from build123d import *

# Parameters (mm, degrees)
BOSS_EXTRUDE1_DEPTH = 28
SKETCH2_W           = 1
SKETCH2_H           = 2
BOSS_EXTRUDE2_DEPTH = 28
SKETCH3_W           = 1
SKETCH3_H           = 2
CUT_EXTRUDE1_DEPTH  = 60.264016753
SKETCH4_R           = 7.5
CUT_EXTRUDE2_DEPTH  = 10
SKETCH5_W           = 1
SKETCH5_H           = 2
CUT_EXTRUDE3_DEPTH  = 10
SKETCH6_W           = 7
SKETCH6_H           = 7.5
CUT_EXTRUDE4_DEPTH  = 2
SKETCH7_W           = 7
SKETCH7_H           = 18.5
CUT_EXTRUDE5_DEPTH  = 1


with BuildPart() as part:
    # Sketch1 → Boss-Extrude1 (new body)
    with BuildSketch(Plane.XY):
        with BuildLine():
            Line((-30.589041096, 0), (-30.589041096, 33))
            ThreePointArc((-30.589041096, 33), (-29.124575002, 36.535533906), (-25.589041096, 38))
            Line((-25.589041096, 38), (19.910958904, 38))
            ThreePointArc((19.910958904, 38), (23.44649281, 36.535533906), (24.910958904, 33))
            Line((24.910958904, 33), (24.910958904, 0))
            Line((24.910958904, 0), (24.910958904, -6))
            Line((24.910958904, -6), (26.910958904, -6))
            Line((26.910958904, -6), (26.910958904, 0))
            Line((26.910958904, 0), (26.910958904, 33))
            ThreePointArc((26.910958904, 33), (24.860706372, 37.949747468), (19.910958904, 40))
            Line((19.910958904, 40), (-25.589041096, 40))
            ThreePointArc((-25.589041096, 40), (-30.538788564, 37.949747468), (-32.589041096, 33))
            Line((-32.589041096, 33), (-32.589041096, 0))
            Line((-32.589041096, 0), (-32.589041096, -6))
            Line((-32.589041096, -6), (-30.589041096, -6))
            Line((-30.589041096, -6), (-30.589041096, 0))
        make_face()
    extrude(amount=BOSS_EXTRUDE1_DEPTH)

    # Sketch2 → Boss-Extrude2 (add, through all)
    with BuildSketch(Plane.XY.offset(28)):
        with Locations((-33.089041096, -5)):
            Rectangle(SKETCH2_W, SKETCH2_H)
        with Locations((27.410958904, -5)):
            Rectangle(SKETCH2_W, SKETCH2_H)
    extrude(amount=-BOSS_EXTRUDE2_DEPTH)

    # Sketch3 → Cut-Extrude1 (cut, through all)
    with BuildSketch(Plane.XY.offset(28)):
        with Locations((-32.089041096, -3)):
            Rectangle(SKETCH3_W, SKETCH3_H)
        with Locations((26.410958904, -3)):
            Rectangle(SKETCH3_W, SKETCH3_H)
    extrude(amount=-CUT_EXTRUDE1_DEPTH, mode=Mode.SUBTRACT)

    # Sketch4 → Cut-Extrude2 (cut)
    with BuildSketch(Plane(origin=(0, 40, 0), x_dir=(1, 0, 0), z_dir=(0, 1, 0))):
        with Locations(Location((4.410958904, -11.6, 0), (0, 0, 270))):
            Circle(SKETCH4_R)
    extrude(amount=-CUT_EXTRUDE2_DEPTH, mode=Mode.SUBTRACT)

    # Sketch5 → Cut-Extrude3 (cut)
    with BuildSketch(Plane(origin=(0, 0, 0), x_dir=(-1, 0, 0), z_dir=(0, 0, -1))):
        with Locations((-27.410958904, -5)):
            Rectangle(SKETCH5_W, SKETCH5_H)
    extrude(amount=-CUT_EXTRUDE3_DEPTH, mode=Mode.SUBTRACT)

    # Sketch6 → Cut-Extrude4 (cut)
    with BuildSketch(Plane(origin=(0, 40, 0), x_dir=(1, 0, 0), z_dir=(0, 1, 0))):
        with Locations((-16.089041096, -5.75)):
            Rectangle(SKETCH6_W, SKETCH6_H)
    extrude(amount=-CUT_EXTRUDE4_DEPTH, mode=Mode.SUBTRACT)

    # Sketch7 → Cut-Extrude5 (cut)
    with BuildSketch(Plane(origin=(0, 40, 0), x_dir=(1, 0, 0), z_dir=(0, 1, 0))):
        with Locations((-16.089041096, -18.75)):
            Rectangle(SKETCH7_W, SKETCH7_H)
    extrude(amount=-CUT_EXTRUDE5_DEPTH, mode=Mode.SUBTRACT)


solid = part.part
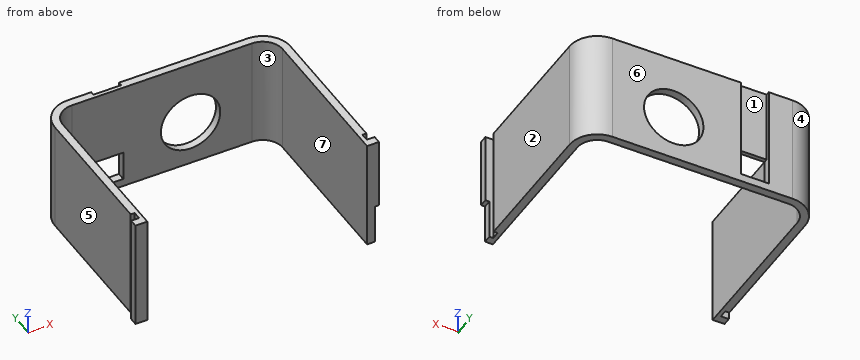
Work out the finished part from the listing and answer in its coordinate system (mm). Face numbers are marked on the shaded views. A direction names the side the tool comes from. Give positions to 0.01 mm unless a question says otherwise; leave off trailing zeros. Order: outer loops, then holes, each group sorted by start corner. A loop starts at its lowest first (then second) coordinate and runs counter-clockwise, first axis right, second up. Notation, with made-up numbers: (-9, 24) -> (25, 24) arc R17 cw to (25, 56) -> close; hole circle Ø10 at (50, 43.25). An arc over 180 degrees is marked (long way). One line per item, written item: value.
Item 1: Find section D-D, the plane z = 25.5. Give the vertices of the cut face in (x, y).
Answer sheet:
outline: (-33.59, -6) -> (-30.59, -6) -> (-30.59, 33) arc R5 cw to (-25.59, 38) -> (19.91, 38) arc R5 cw to (24.91, 33) -> (24.91, -6) -> (27.91, -6) -> (27.91, -4) -> (25.91, -4) -> (25.91, -2) -> (26.91, -2) -> (26.91, 33) arc R7 ccw to (19.91, 40) -> (-12.59, 40) -> (-12.59, 39) -> (-19.59, 39) -> (-19.59, 40) -> (-25.59, 40) arc R7 ccw to (-32.59, 33) -> (-32.59, -2) -> (-31.59, -2) -> (-31.59, -4) -> (-33.59, -4) -> close
Item 2: Find section B-B, the plane x = -17. Give the vertices of the cut face in (y, z), plus the area to 3 significant figures.
Answer sheet:
outline: (38, 0) -> (40, 0) -> (40, 2) -> (38, 2) -> close; (38, 9.5) -> (39, 9.5) -> (39, 28) -> (38, 28) -> close
area: 22.5 mm²
Item 3: Flat-ended cylindrical pins translate along their axes: P1, Ø0.6, axis at y = -2.5, z = 12, coming from the +X side; P2, Ø7.5, axis at x = -16.5, z = 17.5, coming from the +Y side; P3, Ø4, axis at x = 20, z = 15, coming from the -Y side; P4, Ø4, axis at y = 13.5, z = 17, coming from the -X side. Find the tip coordinate at first contact, or state that the pin passes through.
Answer sheet:
P1: x = 25.91
P2: y = 40
P3: y = 37.54
P4: x = -32.59
Item 4: A tool of negligible diameter and unlimited length cuts with its end or side. For the marked faces 5, 6 and 7, from which of +Z, -Z, +X, -X, +Y, -Y can it reach the whole face along a straight path? Write none if from no direction.
Answer sheet:
face 5: +Z, -Z, -X, +Y
face 6: +Z, -Z, +X, -X, +Y
face 7: +Z, -Z, -Y
Item 5: Find section C-C, the plane y = 23.5. Give the vertices of the cut face in (x, z), plus the area to 3 significant figures.
Answer sheet:
outline: (-32.59, 0) -> (-30.59, 0) -> (-30.59, 28) -> (-32.59, 28) -> close; (24.91, 0) -> (26.91, 0) -> (26.91, 28) -> (24.91, 28) -> close
area: 112 mm²
Item 6: Straight lines are drawn through the part: probe 1 along X at (y, z) = (6, 8.5); probe 2 along X at (y, z) = (39.45, 11.6); probe 3 along Y at (x, z) = (-20.5, 2). For each, find the intervals that lie inside material, in ascending order.
Answer sheet:
probe 1: -32.59 to -30.59, 24.91 to 26.91
probe 2: -28.31 to -19.59, -12.59 to -3.09, 11.91 to 22.63
probe 3: 38 to 40
Item 7: Determine the mould class of the marked faces 1, 2, 3 and 4 for opening direction X: released by +X, released by -X, zero draft, split by the parting line, or undercut.
Answer sheet:
face 1: undercut
face 2: released by +X
face 3: undercut
face 4: released by -X
Item 8: Find section A-A, the plane z = 11.6. Give the vertices of the cut face in (x, y).
Answer sheet:
outline: (-33.59, -6) -> (-30.59, -6) -> (-30.59, 33) arc R5 cw to (-25.59, 38) -> (-3.09, 38) -> (-3.09, 40) -> (-12.59, 40) -> (-12.59, 39) -> (-19.59, 39) -> (-19.59, 40) -> (-25.59, 40) arc R7 ccw to (-32.59, 33) -> (-32.59, -2) -> (-31.59, -2) -> (-31.59, -4) -> (-33.59, -4) -> close; (11.91, 38) -> (19.91, 38) arc R5 cw to (24.91, 33) -> (24.91, -6) -> (27.91, -6) -> (27.91, -4) -> (25.91, -4) -> (25.91, -2) -> (26.91, -2) -> (26.91, 33) arc R7 ccw to (19.91, 40) -> (11.91, 40) -> close
